from build123d import *

# Parameters (mm, degrees)
BOSS_EXTRUDE1_DEPTH  = 4.7625
CHAMFER1_SIZE        = 5.3975
CUT_EXTRUDE1_DEPTH   = 2.25
FILLET1_R            = 2.25
FILLET1_OF_MIRROR1_R = 2.25
FILLET2_R            = 3.175
CUT_EXTRUDE2_DEPTH   = 56.557883235
FILLET3_R            = 1.27


# Some blends are built 0.0001 mm under size
with BuildPart() as part:
    # Sketch1 → Boss-Extrude1 (new, symmetric)
    with BuildSketch(Plane(origin=(0, 0, 0), x_dir=(1, 0, 0), z_dir=(0, 1, 0))):
        with BuildLine():
            Line((-19.447559324, 30.526553381), (-21.153485581, 33.204321222))
            ThreePointArc((-21.153485581, 33.204321222), (-15.85613718, 36.035812933), (-10.189705806, 38.028499781))
            Line((-10.189705806, 38.028499781), (-13.065832444, 48.762350526))
            ThreePointArc((-13.065832444, 48.762350526), (0, 50.4825), (13.065832444, 48.762350526))
            Line((13.065832444, 48.762350526), (10.189705806, 38.028499781))
            ThreePointArc((10.189705806, 38.028499781), (15.85613718, 36.035812933), (21.153485581, 33.204321222))
            Line((21.153485581, 33.204321222), (19.447559324, 30.526553381))
            ThreePointArc((19.447559324, 30.526553381), (0, 36.195), (-19.447559324, 30.526553381))
        make_face()
    extrude(amount=BOSS_EXTRUDE1_DEPTH, both=True)

    # Chamfer1
    # the kernel refuses this chamfer: 9.348744234, 5.3975 mm, written as the material it takes off along each edge
    with BuildSketch(Plane(origin=(-13.065832444, 26.081931668, -48.762350526), x_dir=(0.9837865219812311, 0, -0.17934346703482887), z_dir=(0, -1, 0))) as chamfer1_piece_1:
        with BuildLine():
            Line((8.217561706, 0), (CHAMFER1_SIZE * 0.0813902016187, CHAMFER1_SIZE * 0.99668231402))
            Line((CHAMFER1_SIZE * 0.0813902016187, CHAMFER1_SIZE * 0.99668231402), (0, 0))
            ThreePointArc((0, 0), (4.262745394, -0.167250297), (8.217561706, 0))
        make_face()
    extrude(amount=52.163863336, mode=Mode.SUBTRACT)
    with BuildSketch(Plane(origin=(13.065832444, -26.081931668, -48.762350526), x_dir=(-0.25881904510252207, 0, 0.965925826289068), z_dir=(0, 1, 0))) as chamfer1_piece_2:
        with BuildLine():
            Line((CHAMFER1_SIZE, 0), (0.668829004, -8.190298417))
            ThreePointArc((0.668829004, -8.190298417), (0.180250294, -4.262215479), (0, 0))
            Line((0, 0), (CHAMFER1_SIZE, 0))
        make_face()
    extrude(amount=52.163863336, mode=Mode.SUBTRACT)

    # Sketch2 → Cut-Extrude1 (cut, symmetric)
    with BuildSketch(Plane(origin=(0, 0, 0), x_dir=(1, 0, 0), z_dir=(0, 1, 0))):
        with BuildLine():
            Line((-12.165999069, 37.443095047), (-11.184870111, 34.423490607))
            ThreePointArc((-11.184870111, 34.423490607), (-14.577416439, 33.129698987), (-17.823270758, 31.502524415))
            Line((-17.823270758, 31.502524415), (-19.386715561, 34.265903749))
            ThreePointArc((-19.386715561, 34.265903749), (-15.85613718, 36.035812933), (-12.165999069, 37.443095047))
        make_face()
    cut_extrude1 = extrude(amount=CUT_EXTRUDE1_DEPTH, both=True, mode=Mode.SUBTRACT)

    # Fillet1
    fillet1_edges = [part.edges().sort_by_distance(p)[0] for p in [
        (-18.60499316, -2.25, -32.884214082),
        (-18.60499316, 2.25, -32.884214082),
        (-11.67543459, 2.25, -35.933292827),
        (-11.67543459, -2.25, -35.933292827),
    ]]
    fillet(fillet1_edges, radius=FILLET1_R - 0.0001)  # a hair under: the kernel refuses the full size

    # Mirror1: Cut-Extrude1 across plane
    add(cut_extrude1.mirror(Plane(origin=(0, 0, 0), x_dir=(0, 0, 1), z_dir=(1, 0, 0))), mode=Mode.SUBTRACT)

    # Fillet1 of Mirror1
    fillet1_of_mirror1_edges = [part.edges().sort_by_distance(p)[0] for p in [
        (18.60499316, -2.25, -32.884214082),
        (18.60499316, 2.25, -32.884214082),
        (11.67543459, 2.25, -35.933292827),
        (11.67543459, -2.25, -35.933292827),
    ]]
    fillet(fillet1_of_mirror1_edges, radius=FILLET1_OF_MIRROR1_R - 0.0001)  # a hair under: the kernel refuses the full size

    # Fillet2
    fillet2_edges = [part.edges().sort_by_distance(p)[0] for p in [
        (-11.668856648, 0, -43.548765878),
        (4.981505994, 0, -50.236116533),
        (-4.981505994, 0, -50.236116533),
        (11.668856648, 0, -43.548765878),
    ]]
    fillet(fillet2_edges, radius=FILLET2_R)

    # Sketch3 → Cut-Extrude2 (cut, through all)
    with BuildSketch(Plane(origin=(0, 4.7625, 0), x_dir=(1, 0, 0), z_dir=(0, 1, 0))):
        with BuildLine():
            Line((7.089702157, 38.726386655), (8.127604296, 42.59989017))
            Line((8.127604296, 42.59989017), (3.553655431, 47.173839035))
            ThreePointArc((3.553655431, 47.173839035), (0, 47.3075), (-3.553655431, 47.173839035))
            Line((-3.553655431, 47.173839035), (-8.127604296, 42.59989017))
            Line((-8.127604296, 42.59989017), (-7.089702157, 38.726386655))
            ThreePointArc((-7.089702157, 38.726386655), (0, 39.37), (7.089702157, 38.726386655))
        make_face()
    extrude(amount=-CUT_EXTRUDE2_DEPTH, mode=Mode.SUBTRACT)

    # Fillet3
    fillet3_edges = [part.edges().sort_by_distance(p)[0] for p in [
        (7.089702157, 0, -38.726386655),
        (-7.089702157, 0, -38.726386655),
        (-8.127604296, 0, -42.59989017),
        (-3.553655431, 0, -47.173839035),
        (3.553655431, 0, -47.173839035),
        (8.127604296, 0, -42.59989017),
    ]]
    fillet(fillet3_edges, radius=FILLET3_R)


solid = part.part
Design review of the part built by this model. Coordinates are the model's own, in mm. A direction names the side the tool comes from. Give positions to 0.01 mm unless a question says otherwise; leave off trailing zeros. Order: outer loops, then holes, each group sorted by start corner. A loop starts at its lowest first (then second) coordinate and runs counter-clockwise, first axis right, second up. Notation, with made-up numbers: (-18.5, -30.5) - (-4.5, -30.5) arc R26 ccw to (-4.5, 5.5) - close; hole circle Ø11 at (-5.75, -18). An arc over 180 degrees is marked (long way). Use CSV: the item, a comma, the result in double quotes. Start each with the question number.
Q1. Take a section at A-A (y = -1). Count the separate pieces of the cut face and the enclosed holes in it, and give its area (3 significant figures).
Q2. For P1, Ø3, axis at x = 0.5, y = 3.5, coming from the +Z side; P2, Ø2, axis at y = 3, z = -41, coming from the +X side; P3, Ø4, axis at y = -2, z = -40.5, coming from the -X side, all flat-tipped, find the tip position at first contact; note any pin that passes through.
Q3. Take a section at B-B (x = -0.5). State the section outline as (y, z) points.
Q4. Machinability: for faces 5 (the face through (6.867, -0.067, -39.114)), 6 (the face through (-12.3, 1.6, -35.7)), 7 (the face through (-18.041, 1.573, -33.189)), 8 (the face through (15.78, 3.24, -36.07)), 9 (the face through (15, 2.25, -35)), which of the approach directions +Z, -Z, +X, -X, +Y, -Y give a long, thin tool a straight path to every point of the face, cutting with its end or side? Answer none if there is none.
Q5. Draft analysis for pull direction Z (two halves, no side actions). For faces 1 (the face through (-10.685, 0.067, -39.877)), 2 (the face through (7.66, 0.07, -40.85)), 3 (the face through (20.31, 0.07, -31.88)), 4 (the face through (0, -4.762, -39)), state which applies: pulls with the +Z half, pulls with the -Z half, needs draft (parallel to the pull), parting line crosses it, or undercut.
Q6. For line 1 (Z direction, x = -0.5, y = 0.75); line 2 (X direction, y = -2.5, z = -32.25); line 3 (X direction, y = 2.5, z = -46.5), list the stretches that pass through material, from the lowest coordinate up.
Calculated:
1,separate pieces,"3"
1,enclosed holes,"1"
1,area,"199 mm²"
2,P1,"stops at z = -36.14"
2,P2,"stops at x = 11.25"
2,P3,"stops at x = -11.3"
3,outline,"(-4.76, -50.48) - (4.76, -50.48) - (4.76, -47.3) - (-4.76, -47.3) - close; (-4.76, -39.37) - (4.76, -39.37) - (4.76, -36.19) - (-4.76, -36.19) - close"
4,face 5,"+Y, -Y"
4,face 6,"+Z"
4,face 7,"-Z"
4,face 8,"+X, +Y, -Y"
4,face 9,"none"
5,face 1,"undercut"
5,face 2,"undercut"
5,face 3,"pulls with the +Z half"
5,face 4,"needs draft"
6,line 1,"z = -50.48 to -47.3, -39.37 to -36.19"
6,line 2,"x = -20.55 to -16.43, 16.43 to 20.55"
6,line 3,"x = -8.72 to -4.23, 4.23 to 8.72"
